Read the model definition and answer for the solid it produces. Units are mm, in the model's axes. A direction names the side the tool comes from. Coordinates: 2 decimals unless noted, no trailing zeros. Loops run counter-clockwise (first coordinate to the right, second up) from the corner with the lowest first, then second, coordinate; pieces in that order, holes last. Notation, with made-up numbers: (33, 49) -> (74, 49) arc R11 cw to (74, 65) -> close; hole circle Ø7 at (68, -9.5). An arc over 180 degrees is marked (long way). Answer as CSV lines item,"result".
```python
from build123d import *

# Parameters (mm, degrees)
SKETCH1_R           = 2.28
BOSS_EXTRUDE1_DEPTH = 9
SKETCH2_R           = 3
BOSS_EXTRUDE2_DEPTH = 5
CHAMFER1_SIZE       = 0.35


with BuildPart() as part:
    # Sketch1 → Boss-Extrude1 (new body)
    with BuildSketch(Plane(origin=(0, 0, 0), x_dir=(1, 0, 0), z_dir=(0, 1, 0))):
        with Locations(Location((0, 0, 0), (0, 0, 270))):
            Circle(SKETCH1_R)
    extrude(amount=BOSS_EXTRUDE1_DEPTH)

    # Sketch2 → Boss-Extrude2 (add)
    with BuildSketch(Plane(origin=(0, 0, 0), x_dir=(-1, 0, 0), z_dir=(0, -1, 0))):
        with Locations(Location((0, 0, 0), (0, 0, 90))):
            Circle(SKETCH2_R)
    extrude(amount=-BOSS_EXTRUDE2_DEPTH)

    # Chamfer1
    chamfer1_edges = [part.edges().sort_by_distance(p)[0] for p in [
        (0, 5, 3),
    ]]
    chamfer(chamfer1_edges, length=CHAMFER1_SIZE)


solid = part.part
```
Q1. For faces 1 (the face through (-1.4, 7, -1.8)), 2 (the face through (0.9, 2.29, -2.86)), determine the directions among +Z, -Z, +X, -X, +Y, -Y from which every point of the face is accessible in a straight line to the end or side of a thin tool.
Results:
face 1,"+Y"
face 2,"+Y, -Y"
Q2. A cutting plane is placed at D-D, the plane y = 4.75. Write down the section's boundary in (x, z).
Results:
outline,"circle Ø5.8 at (0, 0)"
Q3. A cutting plane is placed at B-B, the plane z = 0. Write down the section's boundary in (x, y).
Results:
outline,"(-3, 0) -> (3, 0) -> (3, 4.65) -> (2.65, 5) -> (2.28, 5) -> (2.28, 9) -> (-2.28, 9) -> (-2.28, 5) -> (-2.65, 5) -> (-3, 4.65) -> close"
Q4. A cutting plane is placed at A-A, the plane x = 0. Write down the section's boundary in (y, z).
Results:
outline,"(0, -3) -> (4.65, -3) -> (5, -2.65) -> (5, -2.28) -> (9, -2.28) -> (9, 2.28) -> (5, 2.28) -> (5, 2.65) -> (4.65, 3) -> (0, 3) -> close"
Q5. A cutting plane is placed at C-C, the plane y = 7.5. Write down the section's boundary in (x, z), and give its area (3 significant figures).
Results:
outline,"circle Ø4.56 at (0, 0)"
area,"16.3 mm²"
Q6. Find the intervals of material crossed by probe 1 along Y at (x, z) = (0.45, 2.3); probe 2 along X at (y, z) = (3.5, 1.95); probe 3 along Z at (x, y) = (1.65, 5.5), in increasing order. Write a range as [from, to].
Results:
probe 1,"y = [0, 5]"
probe 2,"x = [-2.28, 2.28]"
probe 3,"z = [-1.57, 1.57]"
Q7. Given pin 1 Ø1.5 at (x, y) = (-2.5, 7.5) entering from +Z; pin 2 Ø1 at (x, y) = (-0.5, 7) entering from -Z, each flat-ended and moving along its own axis, determine where each tip first touches the part or whether it passes through.
Results:
pin 1,"stops at z = 1.46"
pin 2,"stops at z = -2.28"
